Geometry: see drawing. Coordinates: mm, zero at the bounding-box minimum. Coordinates: 2 decimals unless noted, no trailing zeros. Loops run counter-clockwise (first coordinate to the right, second up) from the corner with the lowest first, then second, coordinate; pieces in that order, holes last. Notation, with made-up numbers: (-34.75, 56) - (-30.75, 56) arc R10 cw to (-30.75, 61) - close; hole circle Ø10 at (33, 33.25). An arc over 180 degrees is marked (long way). Write item = value, one per line. Start each with the question number.
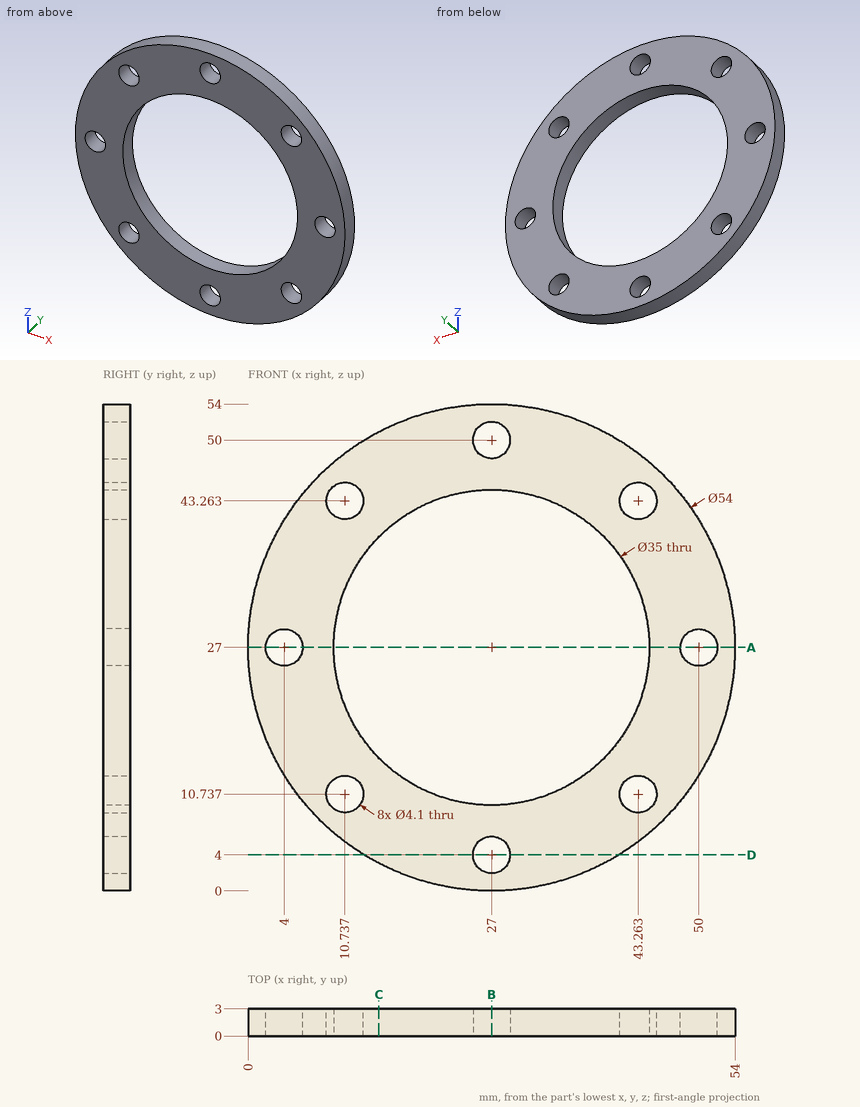
Item 1: Cut plane D-D (z = 4). Return the cut outline in (x, y).
Item 2: Material intervals for L1, parallel to X at y = 1.5, z = 27; L2, parallel to Z at x = 25.5, y = 1.85 (1 decimal); L3, parallel to X at y = 1, z = 42.5 (1 decimal), sorted ascending. Write a range as [from, to].
Item 3: Cut plane C-C (x = 14.5). Return the cut outline in (y, z).
Item 4: Cut plane A-A (z = 27). Return the cut outline in (x, y), then the cut area to 3 significant figures.
Item 5: First-contact query: pin 1 (1.5 mm diameter, centred on x = 25, y = 1.5, fed in from -Z); pin 2 (3.5 mm diameter, centred on x = 43.26, z = 10.74, fed in from +Y). Flat tips, straight axial feed; report the tip coordinate or a pass-through.
Item 6: Cut plane B-B (x = 27). Return the cut outline in (y, z), then the cut area to 3 significant figures.
Responses:
q1.outline = (12.86, 0) - (24.95, 0) - (24.95, 3) - (12.86, 3) - close; (29.05, 0) - (41.14, 0) - (41.14, 3) - (29.05, 3) - close
q2.L1 = [0, 1.95], [6.05, 9.5], [44.5, 47.95], [52.05, 54]
q2.L2 = [0, 2.6], [5.4, 9.6], [44.4, 48.6], [51.4, 54]
q2.L3 = [4.9, 8.8], [12.6, 18.9], [35.1, 41.4], [45.2, 49.1]
q3.outline = (0, 3.07) - (3, 3.07) - (3, 14.75) - (0, 14.75) - close; (0, 39.25) - (3, 39.25) - (3, 50.93) - (0, 50.93) - close
q4.outline = (0, 0) - (1.95, 0) - (1.95, 3) - (0, 3) - close; (6.05, 0) - (9.5, 0) - (9.5, 3) - (6.05, 3) - close; (44.5, 0) - (47.95, 0) - (47.95, 3) - (44.5, 3) - close; (52.05, 0) - (54, 0) - (54, 3) - (52.05, 3) - close
q4.area = 32.4 mm2
q5.pin_1 = 0.03
q5.pin_2 = through
q6.outline = (0, 0) - (3, 0) - (3, 1.95) - (0, 1.95) - close; (0, 6.05) - (3, 6.05) - (3, 9.5) - (0, 9.5) - close; (0, 44.5) - (3, 44.5) - (3, 47.95) - (0, 47.95) - close; (0, 52.05) - (3, 52.05) - (3, 54) - (0, 54) - close
q6.area = 32.4 mm2
